Input: dimensioned drawing with shaded views. Units: mm. Origin: part minimum x, y, z. A direction names the side the tool comes from. Round coordinates to 2 decimals unless told otherwise and drop trailing zeros. Write each loop counter-clockwise with the first axis right and the second up, starting at its lowest first coordinate (ties: lowest second). Pieces come first, ordered by that corner, then holes. Notation, with made-up numbers: M 70.25,10.5 L 98.25,10.5 A11 cw 98.25,23.5 Z; hole C 62.5,-25 d1. An arc over 180 degrees is marked long. Use one line per item in the form item = value. Start each with the question number.
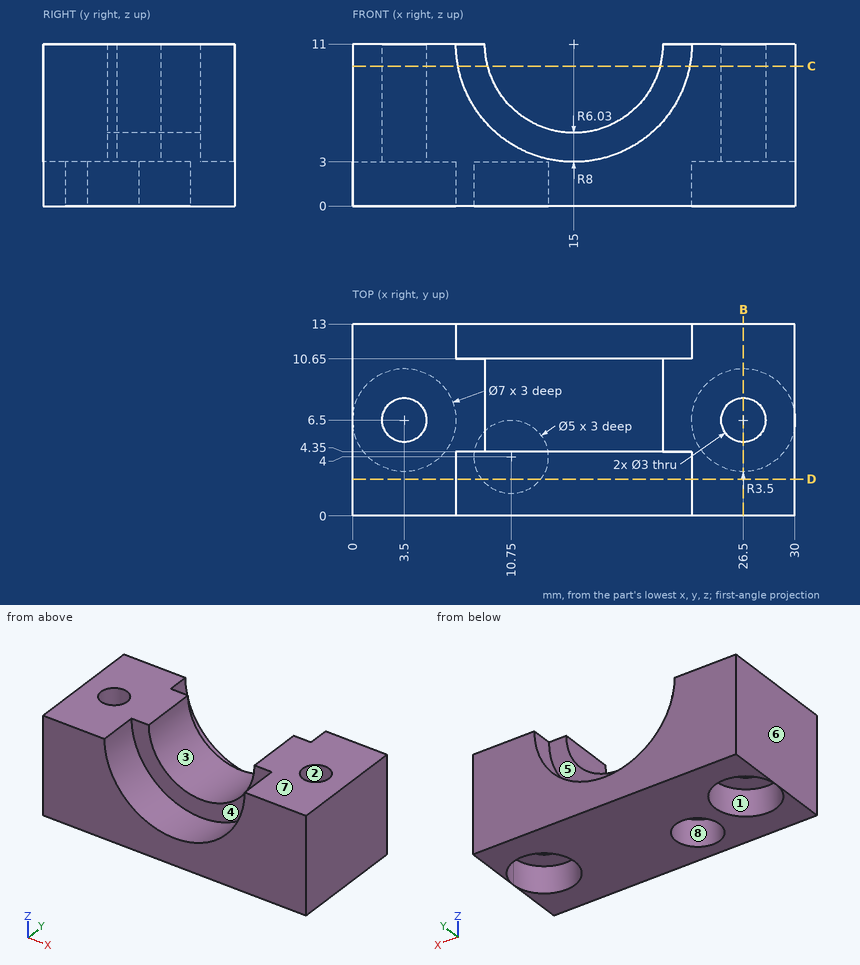
1. Ray query, probe 1 along X at (y, z) = (6.25, 7.5); probe 2 along Y at (x, z) = (3.5, 9.25); probe 3 along X at (y, z) = (8, 0.5). Return the intervals inside material, ascending.
2. Section query C-C (z = 9.5). Return loops of the section in (x, y).
3. Set-up query: the marked faces 1, 2, 3, 4 and 5. Return all of +Z, -Z, +X, -X, +Y, -Y with unobstructed straight access to the full face (end or side cutting, diameter ignored); none if empty.
4. Section query B-B (x = 26.5). Return loops of the section in (y, z), then the cut area to 3 significant figures.
5. Contact query for flat-ended pins moving along their axis: pin 1 (2 mm diameter, centred on x = 3.5, y = 6.5, fed in from -Z); pin 2 (3.5 mm diameter, centred on x = 26.5, y = 6.5, fed in from -Z). Output: stop coordinate, or through.
6. Pull-direction query (X, two-part tool) for the marked faces 6, 7 and 8; classes: released by +X, released by -X, zero draft, split by the parting line, or undercut.
7. Section query D-D (y = 2.5). Return loops of the section in (x, z).
Checks:
q1.probe_1 = 0 to 2.02, 4.98 to 10.09, 19.91 to 25.02, 27.98 to 30
q1.probe_2 = 0 to 5, 8 to 13
q1.probe_3 = 0 to 0.34, 6.66 to 23.34, 29.66 to 30
q2.outline = M 0,0 L 7.14,0 L 7.14,4.35 L 9.16,4.35 L 9.16,10.65 L 7.14,10.65 L 7.14,13 L 0,13 Z; M 20.84,4.35 L 22.86,4.35 L 22.86,0 L 30,0 L 30,13 L 22.86,13 L 22.86,10.65 L 20.84,10.65 Z; hole C 3.5,6.5 d3; hole C 26.5,6.5 d3
q3.face_1 = -Z
q3.face_2 = +Z, -Z
q3.face_3 = +Z, +Y, -Y
q3.face_4 = +Z, -Y
q3.face_5 = +Z, +Y
q4.outline = M 0,0 L 3,0 L 3,3 L 5,3 L 5,11 L 0,11 Z; M 8,3 L 10,3 L 10,0 L 13,0 L 13,11 L 8,11 Z
q4.area = 98.0 mm^2
q5.pin_1 = through
q5.pin_2 = 3
q6.face_6 = released by -X
q6.face_7 = zero draft
q6.face_8 = undercut
q7.outline = M 0,0 L 8.75,0 L 8.75,3 L 12.75,3 L 12.75,0 L 30,0 L 30,11 L 23,11 A8 cw 7,11 L 0,11 Z
